Part model, mm, in its own coordinate system. A direction names the side the tool comes from. Coordinates: 2 decimals unless noted, no trailing zeros. Order: outer loops, then holes, each group sorted by start corner. A loop starts at its lowest first (then second) coordinate and runs counter-clockwise, first axis right, second up. Notation, with made-up numbers: (-7.75, 79.25) - (42.25, 79.25) arc R24 cw to (42.25, 101.25) - close; hole circle Ø10 at (67.5, 73.25). An arc over 180 degrees is marked (long way). Use a Markdown table: item, result. Add a question column.
1) Drop flat-ended pins along their axis: P1, Ø1.5, axis at y = 0, z = 13.5, coming from the -X side (3 decimals); P2, Ø0.5, axis at y = 0, z = 6.5, coming from the +X side. Give the stop position or say it passes through.
2) Saw through at A-A on z = 16.25. List the corners of the cut face in (x, y) (3 decimals).
3) Saw through at B-B on z = 3.25. List the corners of the cut face in (x, y).
4) Tool access for faces 4 (the face through (0, -0.75, 1)), 5 (the face through (0.3, 0.45, 7.6)), 6 (the face through (-1.27, 0, 6)): list every direction of +Z, -Z, +X, -X, +Y, -Y with a clear straight run to the whole face (end or side of a thin tool).
5) Wall check: L1, parallel to Y at x = 0.8, z = 7.75; L2, parallel to Y at x = 1, z = 7.5; L3, parallel to X at y = -0.45, z = 1.5. Give the ranges that are in metal, low to high. Write a range as [from, to].
6) Two-plate mould, pull along X, no slides. Class faces 1 (the face through (0, 0.75, 1)), 2 (the face through (0, -1.27, 6)), 3 (the face through (0.97, 0, 7)): +X half, -X half, draft (parallel to the pull), parting line (faces both ways), or undercut.
Autodesk Fusion 360 part; units mm, degrees
sketch "Sketch1" plane through (0, 0, 0) normal (0, 0, 1) x (1, 0, 0)
  line L0 (1.27, -1.27) -> (-1.27, -1.27)
  line L1 (-1.27, -1.27) -> (-1.27, 1.27)
  line L2 (-1.27, 1.27) -> (1.27, 1.27)
  line L3 (1.27, 1.27) -> (1.27, -1.27)
  line L4 (1.27, -1.27) -> (-1.27, 1.27) construction
  line L5 (-1.27, -1.27) -> (1.27, 1.27) construction
  dimension "d1" = 2.54
  dimension "d2" = 2.54
extrude "Extrude1" add sketch "Sketch1" along normal blind 12
sketch "Sketch2" plane through (0, 0, 12) normal (0, 0, 1) x (-1, 0, 0)
  line L0 (-1.27, -1.27) -> (1.27, -1.27)
  line L1 (1.27, -1.27) -> (1.27, 1.27)
  line L2 (1.27, 1.27) -> (-1.27, 1.27)
  line L3 (-1.27, 1.27) -> (-1.27, -1.27)
  line L4 (-0.45, 0.45) -> (0.45, 0.45)
  line L5 (0.45, 0.45) -> (0.45, -0.45)
  line L6 (0.45, -0.45) -> (-0.45, -0.45)
  line L7 (-0.45, -0.45) -> (-0.45, 0.45)
  line L8 (-0.45, 0.45) -> (0.45, -0.45) construction
  line L9 (0.45, 0.45) -> (-0.45, -0.45) construction
  dimension "d5" = 0.9
  dimension "d6" = 0.9
extrude "Extrude2" cut sketch "Sketch2" against normal blind 0.5 contours L4 L5 L6 L7
loft "Loft1" cut profiles "Sketch2" section 1 section 2 face at (0.15, -0.15, 11.5)
extrude "Extrude3" cut 1 faces at (0.15, -0.15, 11.5) along direction (0, 0, -1) blind 8
sketch "Sketch3" plane through (1.27, 0, 0) normal (1, 0, 0) x (0, 1, 0)
  line L0 (-1.27, 0) -> (1.27, 0)
  line L1 (1.27, 0) -> (1.27, 12)
  line L2 (1.27, 12) -> (-1.27, 12)
  line L3 (-1.27, 12) -> (-1.27, 0)
  line L4 (1, 8) -> (-1, 8)
  line L5 (-1, 8) -> (-1, 2.5)
  line L6 (-1, 2.5) -> (1, 2.5)
  line L7 (1, 2.5) -> (1, 8)
  line L8 (1, 8) -> (-1, 2.5) construction
  line L9 (-1, 8) -> (1, 2.5) construction
  line L10 (0.6482, 2.5061) -> (-0.6518, 2.5061)
  line L11 (-0.6518, 2.5061) -> (-0.6518, 6.0061)
  line L12 (-0.6518, 6.0061) -> (0.6482, 6.0061)
  line L13 (0.6482, 6.0061) -> (0.6482, 2.5061)
  line L14 (0.6482, 2.5061) -> (-0.6518, 6.0061) construction
  line L15 (-0.6518, 2.5061) -> (0.6482, 6.0061) construction
  line L16 (-0.6518, 6.0061) -> (0.6571, 6.0061)
  line L17 (0.6571, 6.0061) -> (0.6571, 8.0061)
  line L18 (0.6571, 8.0061) -> (-0.6518, 8.0061)
  line L19 (-0.6518, 8.0061) -> (-0.6518, 6.0061)
  line L20 (0.5, 6.1311) -> (-0.5, 6.1311)
  line L21 (-0.5, 6.1311) -> (-0.5, 7.8811)
  line L22 (-0.5, 7.8811) -> (0.5, 7.8811)
  line L23 (0.5, 7.8811) -> (0.5, 6.1311)
  line L24 (0.5, 6.1311) -> (-0.5, 7.8811) construction
  line L25 (-0.5, 6.1311) -> (0.5, 7.8811) construction
  line L26 (-1.27, 6) -> (-0.6518, 6.0061)
  line L27 (0.6571, 6.0061) -> (1.27, 6)
  line L28 (0.6482, 2.5061) -> (1, 2.5)
  line L29 (-0.6518, 2.5061) -> (-1, 2.5)
  point P0 (0, 5.25)
  point P1 (-0.0018, 4.2561)
  point P2 (0, 7.0061)
  dimension "d11" = 5.5
  dimension "d12" = 2.5
  dimension "d13" = 1.3
  dimension "d14" = 3.5
  dimension "d15" = 2
  dimension "d16" = 1
  dimension "d17" = 1.75
  dimension "d31" = 0.125
extrude "Extrude4" cut sketch "Sketch3" against normal blind 0.3 contours L5 L11 L26 L29 | L4 L5 L19 L26 | L4 L7 L17 L27 | L7 L13 L16 L27 L28
extrude "Extrude5" cut sketch "Sketch3" against normal blind 0.5 contours L4 L12 L16 L17 L19
extrude "Extrude6" cut sketch "Sketch3" against normal blind 0.3 contours L20 L21 L22 L23
sketch "Sketch4" plane through (0, 0, 0) normal (0, 0, -1) x (1, 0, 0)
  line L0 (-1.27, -1.27) -> (1.27, -1.27)
  line L1 (1.27, -1.27) -> (1.27, 1.27)
  line L2 (1.27, 1.27) -> (-1.27, 1.27)
  line L3 (-1.27, 1.27) -> (-1.27, -1.27)
  line L4 (0.75, -0.75) -> (-0.75, -0.75)
  line L5 (-0.75, -0.75) -> (-0.75, 0.75)
  line L6 (-0.75, 0.75) -> (0.75, 0.75)
  line L7 (0.75, 0.75) -> (0.75, -0.75)
  line L8 (0.75, -0.75) -> (-0.75, 0.75) construction
  line L9 (-0.75, -0.75) -> (0.75, 0.75) construction
  dimension "d24" = 1.5
  dimension "d25" = 1.5
extrude "Extrude7" cut sketch "Sketch4" against normal blind 2 contours L4 L5 L6 L7
sketch "Sketch5" plane through (0, 0, 2) normal (0, 0, -1) x (1, 0, 0)
  line L0 (0.75, 0.75) -> (-0.75, 0.75)
  line L1 (-0.75, 0.75) -> (-0.75, -0.75)
  line L2 (-0.75, -0.75) -> (0.75, -0.75)
  line L3 (0.75, -0.75) -> (0.75, 0.75)
  circle A0 centre (0, 0) radius 0.725
  dimension "d28" = 1.45
extrude "Extrude8" add sketch "Sketch5" along normal blind 0.1 contours A0
sketch "Sketch6" plane through (0, 0, 3.5) normal (0, 0, 1) x (-1, 0, 0)
  line L0 (-0.45, -0.45) -> (0.45, -0.45)
  line L1 (0.45, -0.45) -> (0.45, 0.45)
  line L2 (0.45, 0.45) -> (-0.45, 0.45)
  line L3 (-0.45, 0.45) -> (-0.45, -0.45)
  line L4 (-0.325, 0.325) -> (0.325, 0.325)
  line L5 (0.325, 0.325) -> (0.325, -0.325)
  line L6 (0.325, -0.325) -> (-0.325, -0.325)
  line L7 (-0.325, -0.325) -> (-0.325, 0.325)
  line L8 (-0.325, 0.325) -> (0.325, -0.325) construction
  line L9 (0.325, 0.325) -> (-0.325, -0.325) construction
  dimension "d32" = 0.65
  dimension "d33" = 0.65
extrude "Extrude9" add sketch "Sketch6" along normal blind 14.5 contours L4 L5 L6 L7
fillet "Fillet1" radius 0.2 8 edges at (0.325, -0.325, 10.75) (-0.325, -0.325, 10.75) (0.325, 0.325, 10.75) (-0.325, 0.325, 10.75) (-0.325, 0, 18) (0, 0.325, 18) (0.325, 0, 18) (0, -0.325, 18)
equation "d34 = 8.50 mm + 6 mm"
Results are:
| question | item | result |
|---|---|---|
| 1 | P1 | x = -0.325 |
| 1 | P2 | x = 0.97 |
| 2 | outline | (-0.325, -0.125) arc R0.2 ccw to (-0.125, -0.325) - (0.125, -0.325) arc R0.2 ccw to (0.325, -0.125) - (0.325, 0.125) arc R0.2 ccw to (0.125, 0.325) - (-0.125, 0.325) arc R0.2 ccw to (-0.325, 0.125) - close |
| 3 | outline | (-1.27, -1.27) - (1.27, -1.27) - (1.27, -1) - (0.97, -1) - (0.97, -0.65) - (1.27, -0.65) - (1.27, 0.65) - (0.97, 0.65) - (0.97, 1) - (1.27, 1) - (1.27, 1.27) - (-1.27, 1.27) - close |
| 4 | face 4 | -Z |
| 4 | face 5 | +Z |
| 4 | face 6 | +Z, -Z, -X, +Y, -Y |
| 5 | L1 | [-1.27, -0.65], [-0.5, 0.5], [0.66, 1.27] |
| 5 | L2 | [-1.27, -1], [1, 1.27] |
| 5 | L3 | [-1.27, -0.75], [0.75, 1.27] |
| 6 | face 1 | undercut |
| 6 | face 2 | draft |
| 6 | face 3 | +X half |
